The listing builds one solid part. Answer for the finished solid, in the listing's coordinates (mm). A direction names the side the tool comes from. Give positions to 0.01 mm unless a question says otherwise; leave off trailing zeros. Order: outer loops, then holes, each group sorted by start corner. A loop starts at its lowest first (then second) coordinate and runs counter-clockwise, first axis right, second up. Notation, with made-up numbers: (61.5, 71.5) - (99.5, 71.5) arc R20 ccw to (99.5, 85.5) - close; hole circle Ø8 at (89, 1). An arc over 180 degrees is marked (long way). Answer in a Markdown table with one row per item.
from build123d import *

# Parameters (mm, degrees)
F3_DEPTH        = 254.2296
F3_COPIES_COUNT = 30
F6_DEPTH        = 5
F7_SIZE         = 1.016


# Not quite as in the source:
# - a pattern or mirror of a feature is missing from the dataset's text; its kind, count and spacing are read off the source's solid


with BuildPart() as f1:
    # F0 (on Right) → F1 (revolve)
    with BuildSketch(Plane.YZ):
        Polygon((59.2582, 23.876), (0, 23.876), (0, 27.1526), (-114.3, 27.1526), (-114.3, 23.876), (-129.54, 23.876), (-129.54, 20.6375), (-213.4616, 20.6375), (-213.4616, 17.5006), (-233.934, 17.5006), (-233.934, 6.985), (-237.236, 6.985), (-237.236, 3.99415), (-240.2332, 3.99415), (-240.2332, 3.3655), (-248.9962, 3.3655), (-250.0850537402, 3.99415), (-254.2286, 3.99415), (-254.2286, 0), (-233.934, 0), (183.4388, 0), (183.4388, 18.9992), (103.4288, 18.9992), (103.4288, 19.9898), (59.2582, 19.9898), align=None)
    revolve(axis=Axis((0, -25.2476, 0), (0, 1, 0)))

    # F2 (on face) → F3 (cut, through all)
    with BuildSketch(Plane(origin=(0, 0, 0), x_dir=(-1, 0, 0), z_dir=(0, 1, 0))):
        with BuildLine():
            Line((-0.442078818, 26.3868970263), (0, 27.1526))
            ThreePointArc((0, 27.1526), (-2.8382195517, 27.0038552162), (-5.6453429761, 26.5592505437))
            Line((-5.6453429761, 26.5592505437), (-5.0537260411, 25.9021933716))
            ThreePointArc((-5.0537260411, 25.9021933716), (-2.7585688627, 26.2460295319), (-0.442078818, 26.3868970263))
        make_face()
    f3 = extrude(amount=-F3_DEPTH, mode=Mode.SUBTRACT)

    # F3_copies: F3 ×30 about axis
    f3_copies_axis = Axis((0, 0, 0), (0, 1, 0))
    for i in range(1, F3_COPIES_COUNT):
        add(f3.rotate(f3_copies_axis, i * 360 / F3_COPIES_COUNT), mode=Mode.SUBTRACT)

    # F5 (on offset) → F6 (cut)
    with BuildSketch(Plane.XY.offset(18.9992)):
        Polygon((-4.99999, 174.4472), (-4.99999, 113.4872), (4.99999, 113.4872), (4.99999, 174.4472), (0, 174.4472), align=None)
    extrude(amount=-F6_DEPTH, mode=Mode.SUBTRACT)

    # F7
    f7_edges = [f1.edges().sort_by_distance(p)[0] for p in [
        (0, 183.4388, -18.9992),
        (0, -233.934, -17.5006),
    ]]
    chamfer(f7_edges, length=F7_SIZE)


solid = f1.part
Item 1: Consider line 1 (Y direction, x = 2, z = -15.5); line 2 (Y direction, x = 5, z = -17); line 3 (X direction, y = -28, z = 17). Determine where each line is inside the solid, lowest interval first.
Answer block:
| item | result |
|---|---|
| line 1 | -233.93 to 183.44 |
| line 2 | -213.46 to 183.44 |
| line 3 | -20.19 to 20.19 |
Item 2: Find section C-C on y = 83. Write down the section's boundary in (x, z), then the cut area to 3 significant figures.
Answer block:
| item | result |
|---|---|
| outline | circle Ø39.98 at (0, 0) |
| area | 1,260 mm² |
Item 3: Each of these flat-tipped pins is pushed along its axis until it touches: P1, Ø10, axis at x = -20.5, y = -59.5, coming from the -Z side; P2, Ø1.3, axis at y = 153, z = 16.5, coming from the -X side; P3, Ø5, axis at y = 58, z = -20, coming from the +X side. Where does it stop, or does it pass through?
Answer block:
| item | result |
|---|---|
| P1 | z = -21.97 |
| P2 | x = -10.48 |
| P3 | x = 16.24 |
Item 4: Find section A-A on y = -179. Write down the section's boundary in (x, z) (1 decimal).
Answer block:
| item | result |
|---|---|
| outline | circle Ø41.3 at (0, 0) |
Item 5: Find section B-B on y = 157.5. Write down the section's boundary in (x, z), then the cut area to 3 significant figures.
Answer block:
| item | result |
|---|---|
| outline | (-5, 14) - (-5, 18.33) arc R19 ccw (long way) to (5, 18.33) - (5, 14) - close |
| area | 1,090 mm² |
Item 6: Which of the six approach directions +Z, -Z, +X, -X, +Y, -Y give full straight-line access (tool end or side, diameter ignored) to faces 4 (the face through (6, 81.03, 19.07)), 5 (the face through (5.26, -223.33, 16.69))?
Answer block:
| item | result |
|---|---|
| face 4 | +Y |
| face 5 | -Y |
Item 7: Determine the mould class of faces 1 (the face through (-2.05, -244.68, -2.67)), 2 (the face through (-15.2, -213.462, -9.3)), 3 (the face through (-7, 103.429, -18)) for opening direction Y: pulls with the +Y half, pulls with the -Y half, needs draft (parallel to the pull), parting line crosses it, or undercut.
Answer block:
| item | result |
|---|---|
| face 1 | undercut |
| face 2 | pulls with the -Y half |
| face 3 | pulls with the +Y half |
